Design review of the part built by this model. Coordinates are the model's own, in mm. A direction names the side the tool comes from. Round coordinates to 2 decimals unless told otherwise and drop trailing zeros. Write each loop counter-clockwise with the first axis right and the second up, starting at its lowest first coordinate (ties: lowest second). Pieces come first, ordered by that corner, then holes. Notation, with made-up numbers: (23.25, 50) - (74.25, 50) arc R13 ccw to (74.25, 67) - close; hole circle Ø2 at (12.5, -21). An arc over 180 degrees is marked (long way). Use one line per item in the form item = value.
```python
from build123d import *

# Parameters (mm, degrees)
SKETCH1_W                      = 71.12
SKETCH1_H                      = 71.12
BOSS_EXTRUDE1_DEPTH            = 12.7
SKETCH2_R                      = 38.1
CUT_EXTRUDE1_DEPTH             = 8.89
F_7_0_201_DIAMETER_HOLE1_D     = 5.1054
F_7_0_201_DIAMETER_HOLE1_DEPTH = 31.75
F_7_0_201_DIAMETER_HOLE1_TIP   = 1.533816902


with BuildPart() as part:
    # Sketch1 → Boss-Extrude1 (new body)
    with BuildSketch(Plane.XY):
        Rectangle(SKETCH1_W, SKETCH1_H)
    extrude(amount=BOSS_EXTRUDE1_DEPTH)

    # Sketch2 → Cut-Extrude1 (cut)
    with BuildSketch(Plane(origin=(0, 0, 0), x_dir=(-1, 0, 0), z_dir=(0, 0, -1))):
        Circle(SKETCH2_R)
    extrude(amount=-CUT_EXTRUDE1_DEPTH, mode=Mode.SUBTRACT)

    # #7 (0.201) Diameter Hole1
    with Locations(Plane.XY.offset(12.7)):
        with Locations((30.48, 30.48), (-30.48, 30.48), (-30.48, -30.48), (30.48, -30.48)):
            Hole(F_7_0_201_DIAMETER_HOLE1_D / 2, depth=F_7_0_201_DIAMETER_HOLE1_DEPTH)
            with Locations((0, 0, -(F_7_0_201_DIAMETER_HOLE1_DEPTH + F_7_0_201_DIAMETER_HOLE1_TIP / 2))):  # 118° drill point
                Cone(0, F_7_0_201_DIAMETER_HOLE1_D / 2, F_7_0_201_DIAMETER_HOLE1_TIP, mode=Mode.SUBTRACT)


solid = part.part
```
Q1. To check wall thickness, follow line 1 along X through (y, z) = (-19, 6.25); line 2 along Y through (x, z) = (32.5, 3.25); line 3 along X through (y, z) = (-31, 2.5). State the ranges of each line that lie inside material, in increasing order. Write a range as from..to.
Calculated:
line_1 = -35.56..-33.02, 33.02..35.56
line_2 = -35.56..-32.04, -28.92..-19.88, 19.88..28.92, 32.04..35.56
line_3 = -35.56..-32.98, -27.98..-22.15, 22.15..27.98, 32.98..35.56
Q2. Draft analysis for pull direction Y (two halves, no side actions). For faces 3 (the flat face through (-0.5, 35.56, 9.1)), 4 (the flat face through (-0.5, -35.56, 9.1)), 5 (the flat face through (29, -28, 0)), 6 (the cylindrical face through (28.122, 29.502, 6.261)), state which applies: released by +Y, released by -Y, zero draft, split by the parting line, or undercut.
Calculated:
face_3 = released by +Y
face_4 = released by -Y
face_5 = zero draft
face_6 = undercut
Q3. We need section D-D on z = 11.75. Write out the cut boundary in (x, y), then the cut area to 3 significant figures.
Calculated:
outline = (-35.56, -35.56) - (35.56, -35.56) - (35.56, 35.56) - (-35.56, 35.56) - close; hole circle Ø5.11 at (-30.48, -30.48); hole circle Ø5.11 at (-30.48, 30.48); hole circle Ø5.11 at (30.48, -30.48); hole circle Ø5.11 at (30.48, 30.48)
area = 4,980 mm2
Q4. We need section B-B on z = 6.5. Write out the cut boundary in (x, y), then the cut area to 3 significant figures.
Calculated:
outline = (-35.56, -35.56) - (-13.68, -35.56) arc R38.1 cw to (-35.56, -13.68) - close; (-35.56, 13.68) arc R38.1 cw to (-13.68, 35.56) - (-35.56, 35.56) - close; (13.68, -35.56) - (35.56, -35.56) - (35.56, -13.68) arc R38.1 cw to start; (13.68, 35.56) arc R38.1 cw to (35.56, 13.68) - (35.56, 35.56) - close; hole circle Ø5.11 at (-30.48, -30.48); hole circle Ø5.11 at (-30.48, 30.48); hole circle Ø5.11 at (30.48, -30.48); hole circle Ø5.11 at (30.48, 30.48)
area = 602 mm2
Q5. Machinability: for faces 1 (the flat face through (-28, -29, 0)), 2 (the cylindrical face through (27.1, -26.78, 4.38)), which of the approach directions +Z, -Z, +X, -X, +Y, -Y give a long, thin tool a straight path to every point of the face, cutting with its end or side? Answer none if there is none.
Calculated:
face_1 = -Z, +X, -X, +Y, -Y
face_2 = -Z
Q6. For P1, Ø5, axis at x = 10.5, y = 16, coming from the -Z side; P2, Ø3, axis at x = 30.48, y = 30.48, coming from the +Z side, all flat-tipped, find the tip position at first contact; note any pin that passes through.
Calculated:
P1 = 8.89
P2 = through
Q7. We need section A-A on x = -30.48. Write out the cut boundary in (y, z).
Calculated:
outline = (-35.56, 0) - (-33.03, 0) - (-33.03, 12.7) - (-35.56, 12.7) - close; (-27.93, 0) - (-22.86, 0) - (-22.86, 8.89) - (22.86, 8.89) - (22.86, 0) - (27.93, 0) - (27.93, 12.7) - (-27.93, 12.7) - close; (33.03, 0) - (35.56, 0) - (35.56, 12.7) - (33.03, 12.7) - close
